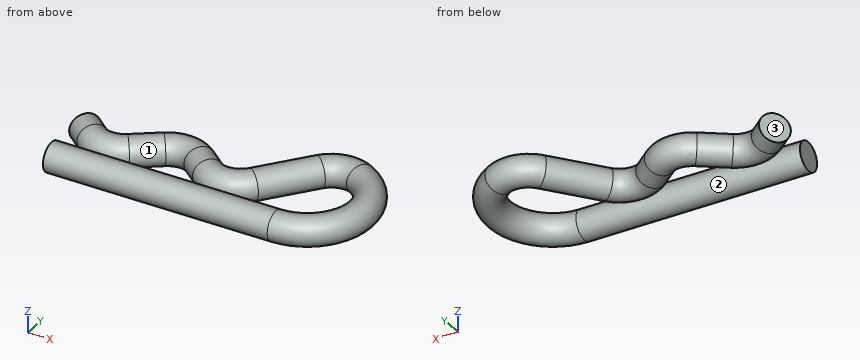
from build123d import *

# Parameters (mm, degrees)
SKETCH2_R = 4.9


with BuildPart() as part:
    # Sweep1: sweep along a path in Sketch1
    with BuildLine(Plane.XY) as sweep1_path:
        Line((0, 0), (75, 0))
        ThreePointArc((75, 0), (92.622639779, 13.738596191), (83.598269269, 34.180396379))
        ThreePointArc((83.598269269, 34.180396379), (76.966606242, 35.188525158), (71.189841712, 31.779086834))
        Line((71.189841712, 31.779086834), (58.000779789, 15.97968974))
        ThreePointArc((58.000779789, 15.97968974), (51.220886684, 12.428395153), (43.915633809, 14.711359059))
        Line((43.915633809, 14.711359059), (38.376494478, 19.33533624))
        ThreePointArc((38.376494478, 19.33533624), (32.391635437, 21.649624212), (26.232382515, 19.8501604))
        Line((26.232382515, 19.8501604), (17.603773383, 13.808437509))
        ThreePointArc((17.603773383, 13.808437509), (11.444520462, 12.008973698), (5.45966142, 14.32326167))
        Line((5.45966142, 14.32326167), (0.509042861, 18.455951945))
    # Sketch2 → Sweep1 (sweep)
    with BuildSketch(Plane(origin=(0, 0, 0), x_dir=(0, 0, -1), z_dir=(1, 0, 0))):
        Circle(SKETCH2_R)
    sweep(path=sweep1_path.line)


solid = part.part
The listing builds one solid part. Answer for the finished solid, in the listing's coordinates (mm). Face numbers are marked on the shaded views. Coordinates: 2 decimals unless noted, no trailing zeros. Loops run counter-clockwise (first coordinate to the right, second up) from the corner with the lowest first, then second, coordinate; pieces in that order, holes last.
1) Determine the mould class of the marked faces 1, 2 and 3 for opening direction X: pulls with the +X half, pulls with the -X half, needs draft (parallel to the pull), parting line crosses it, or undercut.
2) Find section B-B on y = 17. Give the number of separate pieces and of enclosed holes in the cut face, then the cut area to 3 significant figures.
3) Find the intervals of material crossed by L1, parallel to X at y = 10.5, z = 2.5; L2, parallel to X at y = 21, z = -2.75; L3, parallel to X at y = 12, z = -3.5, in increasing order.
4) Find section A-A on z = 0. Write down the section's boundary in (x, y).
5) Flat-ended cylindrical pins translate along their axes: pin 1 Ø3 at (x, z) = (23, -2.5) entering from -Y; pin 2 Ø1 at (x, y) = (48, 8) entering from +Z; pin 3 Ø5 at (y, z) = (4.5, -1) entering from -X. Find the tip coordinate at first contact, or state that the pin passes through.
Values:
1. face 1: undercut
1. face 2: needs draft
1. face 3: pulls with the -X half
2. separate pieces: 3
2. enclosed holes: 0
2. area: 547 mm2
3. L1: x = 3.51 to 20.23, 42.53 to 58.12, 86.66 to 96.03
3. L2: x = 2.63 to 3.79, 20.8 to 42.71, 56.91 to 67.47, 88.83 to 97.05
3. L3: x = 2.89 to 21, 41.81 to 58.83, 88.39 to 95.7
4. outline: (-2.63, 14.69) - (2.32, 10.56) arc R14.9 ccw to (20.41, 9.79) - (29.04, 15.84) arc R5.1 cw to (35.24, 15.57) - (40.78, 10.95) arc R14.9 ccw to (61.76, 12.84) - (74.95, 28.64) arc R5.1 cw to (81.28, 29.86) arc R13.27 cw to (75, 4.9) - (0, 4.9) - (0, -4.9) - (75, -4.9) arc R23.07 ccw to (85.92, 38.5) arc R14.9 ccw to (67.43, 34.92) - (54.24, 19.12) arc R5.1 cw to (47.06, 18.47) - (41.52, 23.1) arc R14.9 ccw to (23.42, 23.86) - (14.79, 17.82) arc R5.1 cw to (8.6, 18.08) - (3.65, 22.22) - close
5. pin 1: stops at y = -4.8
5. pin 2: stops at z = 2.72
5. pin 3: stops at x = 0
